Print and shaded views of the part. All mm, measured from the part's lowest x, y and z. A direction names the side the tool comes from. Round coordinates to 2 decimals unless told otherwise and drop trailing zeros. Order: outer loops, then holes, each group sorted by start corner. A loop starts at its lowest first (then second) coordinate and runs counter-clockwise, first axis right, second up. Notation, with made-up numbers: M 32,53.25 L 54,53.25 A20 ccw 54,71.25 Z; hole C 61,-32.5 d11. An arc over 180 degrees is marked long. Use CSV: the item, a comma, the result in double quotes.
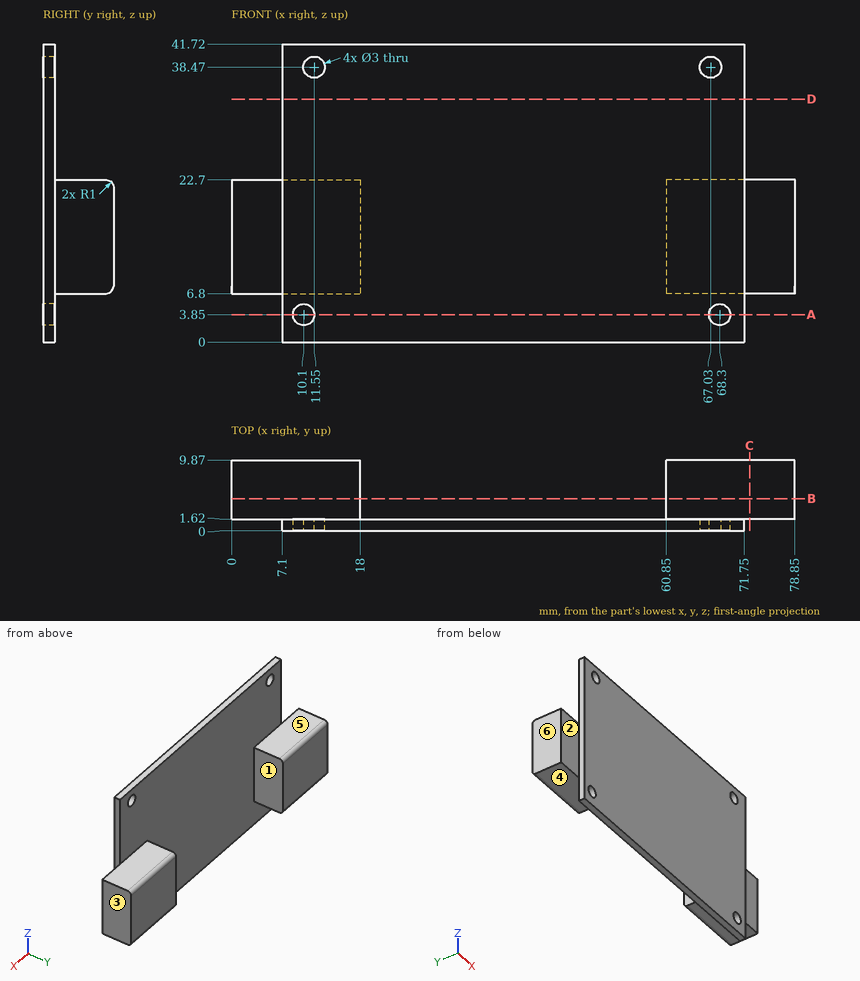
(1) Two-plate mould, pull along X, no slides. Class the marked faces 1, 2 and 3: released by +X, released by -X, zero draft, split by the parting line, or undercut.
Answer block:
face 1,"undercut"
face 2,"zero draft"
face 3,"released by +X"
(2) Tool access for the marked faces 4, 5 and 6: list every direction of +Z, -Z, +X, -X, +Y, -Y with a clear straight run to the whole face (end or side of a thin tool).
Answer block:
face 4,"-Z, +X, -X, +Y"
face 5,"+Z, +X, -X, +Y"
face 6,"+Z, -Z, -X, +Y, -Y"
(3) Wall check: line 1 (X direction, y = 0.8, z = 38.47); line 2 (X direction, y = 1.3, z = 3.85); line 3 (Z direction, x = 67.03, y = 1.2). Give the ranges that are in metal, low to high. Write a range as from..to.
Answer block:
line 1,"x = 7.1..10.05, 13.05..65.53, 68.53..71.75"
line 2,"x = 7.1..8.6, 11.6..66.8, 69.8..71.75"
line 3,"z = 0..3.05, 4.65..36.97, 39.97..41.72"
(4) Cut at D-D, the plane z = 34. Give the cut face in (x, y).
Answer block:
outline,"M 7.1,0 L 71.75,0 L 71.75,1.62 L 7.1,1.62 Z"
(5) Cut at C-C, the plane x = 72.5. Give the cut face in (y, z), and give its area (3 significant figures).
Answer block:
outline,"M 1.62,6.8 L 8.87,6.8 A1 ccw 9.87,7.8 L 9.87,21.7 A1 ccw 8.87,22.7 L 1.62,22.7 Z"
area,"131 mm²"
(6) Cut at B-B, the plane y = 4.5. Give the cut face in (x, z), and give its area (3 significant figures).
Answer block:
outline,"M 0,6.8 L 18,6.8 L 18,22.7 L 0,22.7 Z; M 60.85,6.8 L 78.85,6.8 L 78.85,22.7 L 60.85,22.7 Z"
area,"572 mm²"
(7) Cut at A-A, the plane z = 3.85. Give the cut face in (x, y), and give its area (3 significant figures).
Answer block:
outline,"M 7.1,0 L 8.6,0 L 8.6,1.62 L 7.1,1.62 Z; M 11.6,0 L 66.8,0 L 66.8,1.62 L 11.6,1.62 Z; M 69.8,0 L 71.75,0 L 71.75,1.62 L 69.8,1.62 Z"
area,"95.0 mm²"
(8) Drop flat-ended pins along their axis: pin 1 (3.5 mm diameter, centred on x = 2.5, z = 15, fed in from -Y); pin 2 (5 mm diameter, centred on x = 67.03, z = 38.47, fed in from +Y); pin 3 (3.5 mm diameter, centred on x = 10, y = 6, fed in from +Z). Give the stop position or say it passes through.
Answer block:
pin 1,"stops at y = 1.62"
pin 2,"stops at y = 1.62"
pin 3,"stops at z = 22.7"
